Check sheet for the modelled part. Datum: model origin and axes. Units: mm. Face numbers are marked on the shaded views. A direction names the side the tool comes from. Coordinates: 2 decimals unless noted, no trailing zeros. Order: outer loops, then holes, each group sorted by start corner. A loop starts at its lowest first (then second) coordinate and runs counter-clockwise, first axis right, second up.
from build123d import *

# Parameters (mm, degrees)
SKETCH1_R           = 3.175
BOSS_EXTRUDE1_DEPTH = 95.25


with BuildPart() as part:
    # Sketch1 → Boss-Extrude1 (new body, symmetric)
    with BuildSketch(Plane(origin=(0, 0, 0), x_dir=(1, 0, 0), z_dir=(0, 1, 0))):
        with BuildLine():
            ThreePointArc((20.648095119, -3.175), (31.115, 0), (20.648095119, 3.175))
            Line((20.648095119, 3.175), (-20.648095119, 3.175))
            ThreePointArc((-20.648095119, 3.175), (-31.115, 0), (-20.648095119, -3.175))
            Line((-20.648095119, -3.175), (20.648095119, -3.175))
        make_face()
        with Locations((-25.4, 0)):
            Circle(SKETCH1_R, mode=Mode.SUBTRACT)
        with Locations((25.4, 0)):
            Circle(SKETCH1_R, mode=Mode.SUBTRACT)
    extrude(amount=BOSS_EXTRUDE1_DEPTH, both=True)


solid = part.part
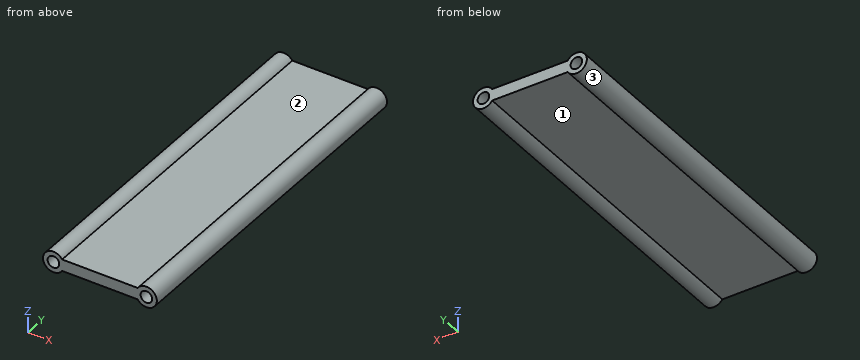
(1) Cross-section at C-C (y = 77.5). Enter the section's corners in (x, z) (3 decimals).
Filled in:
outline: (-20.648, -3.175) - (20.648, -3.175) arc R5.715 ccw (long way) to (20.648, 3.175) - (-20.648, 3.175) arc R5.715 ccw (long way) to start; hole circle Ø6.35 at (-25.4, 0); hole circle Ø6.35 at (25.4, 0)
(2) Tool access check on the marked faces 1, 2 and 3. Record the directions out of +Z, -Z, +X, -X, +Y, -Y that give a thin tool (end or side, any length) a straight path to the whole face; none if there is none.
Filled in:
face 1: -Z, +Y, -Y
face 2: +Z, +Y, -Y
face 3: +Y, -Y
(3) Go/stop test with a flat-tipped pin: P1, Ø1.5, axis at x = -1, y = -20, coming from the +Z side (3 decimals). Record where the tip stops, or that it passes through.
Filled in:
P1: stops at z = 3.175
(4) Cross-section at B-B (z = 0). Enter the section's corners in (x, y) (3 decimals).
Filled in:
outline: (-31.115, -95.25) - (-28.575, -95.25) - (-28.575, 95.25) - (-31.115, 95.25) - close; (-22.225, -95.25) - (22.225, -95.25) - (22.225, 95.25) - (-22.225, 95.25) - close; (28.575, -95.25) - (31.115, -95.25) - (31.115, 95.25) - (28.575, 95.25) - close
(5) Cross-section at A-A (x = -25.4). Enter the section's corners in (y, z) (3 decimals).
Filled in:
outline: (-95.25, -5.715) - (95.25, -5.715) - (95.25, -3.175) - (-95.25, -3.175) - close; (-95.25, 3.175) - (95.25, 3.175) - (95.25, 5.715) - (-95.25, 5.715) - close
(6) Thickness scan on probe 1 along X at (y, z) = (27, 0) (3 decimals); probe 2 along X at (y, z) = (46.5, 0.5); probe 3 along Z at (x, y) = (-25.4, -33.5) (3 decimals). Record the ranges inside material, lowest first.
Filled in:
probe 1: x = -31.115 to -28.575, -22.225 to 22.225, 28.575 to 31.115
probe 2: x = -31.09 to -28.54, -22.26 to 22.26, 28.54 to 31.09
probe 3: z = -5.715 to -3.175, 3.175 to 5.715
(7) Cross-section at D-D (x = 6.5). Enter the section's corners in (y, z) (3 decimals), and give its area (3 significant figures).
Filled in:
outline: (-95.25, -3.175) - (95.25, -3.175) - (95.25, 3.175) - (-95.25, 3.175) - close
area: 1,210 mm2
